Source: CAD feature listing. Evaluate the final solid. Frame: model axes, mm. A direction names the side the tool comes from. Round coordinates to 2 decimals unless told otherwise and drop trailing zeros. Write each loop counter-clockwise with the first axis right and the second up, starting at its lowest first coordinate (ties: lowest second). Pieces come first, ordered by that corner, then holes. Notation, with made-up numbers: (34.25, 50.5) -> (40.25, 50.5) arc R4 cw to (40.25, 56.5) -> close; hole circle Ø7 at (-19.75, -7.75). An arc over 180 degrees is marked (long way). Put each result on its own line as item: value.
```python
from build123d import *

# Parameters (mm, degrees)
PAD_DEPTH        = 11.43
MIRRORED_FACE5_W = 11.43
MIRRORED_FACE5_H = 20.32
PAD001_DEPTH     = 6.85
SKETCH001_W      = 4.191
SKETCH001_H      = 1.778
POCKET_DEPTH     = 10.16
CHAMFER_SIZE     = 1


with BuildPart() as part:
    # Sketch → Pad (new body)
    with BuildSketch(Plane.XZ):
        with BuildLine():
            Line((0, 0), (-10.16, 0))
            add(Edge.make_bspline(
                [(-10.16, 0), (-10.491854, 4.757151), (-8.764645, 7.62), (-8.764645, 7.62)],
                knots=[0, 0, 0, 0, 1, 1, 1, 1], degree=3))
            add(Edge.make_bspline(
                [(-8.764645, 7.62), (-6.92736, 3.81), (0, 3.81)],
                knots=[0, 0, 0, 1, 1, 1], degree=2))
            Line((0, 3.81), (0, 0))
        make_face()
    extrude(amount=PAD_DEPTH)

    # Mirrored: part across YZ


with BuildPart() as part_1:
    add(part.part)
    add(part.part.mirror(Plane.YZ))

    # Mirrored Face5 → Pad001 (add)
    with BuildSketch(Plane(origin=(0, -5.715, 0), x_dir=(0, -1, 0), z_dir=(0, 0, -1))):
        Rectangle(MIRRORED_FACE5_W, MIRRORED_FACE5_H)
    extrude(amount=PAD001_DEPTH)

    # Sketch001 (on Face4 of Pad001) → Pocket (cut)
    with BuildSketch(Plane(origin=(0, 0, -6.85), x_dir=(1, 0, 0), z_dir=(0, 0, -1))):
        with Locations((0, 5.715)):
            Rectangle(SKETCH001_W, SKETCH001_H)
    extrude(amount=-POCKET_DEPTH, mode=Mode.SUBTRACT)

    # Chamfer
    chamfer_edges = [part_1.edges().sort_by_distance(p)[0] for p in [
        (0, 0, -6.85),
        (10.16, -5.715, -6.85),
        (0, -11.43, -6.85),
        (-10.16, -5.715, -6.85),
    ]]
    chamfer(chamfer_edges, length=CHAMFER_SIZE)


solid = part_1.part
```
Q1. Reachability of faces 5 (the flat face through (0, -11.43, -1)), 6 (the flat face through (2.096, -6, -2)), 7 (the flat face through (-10.16, -6, -3)) from +Z, -Z, +X, -X, +Y, -Y: full face, straight path, thin tool, end or side. Return the list, or none.
Ans:
face 5: +Z, -Z, +X, -X, -Y
face 6: -Z
face 7: -Z, -X, +Y, -Y
Q2. Material intervals for line 1 (Y direction, x = 1.25, z = 0.25); line 2 (X direction, y = -3.5, z = -2.25); line 3 (X direction, y = -5, z = 0.5), sorted ascending. Write a range as [from, to].
Ans:
line 1: y = [-11.43, -6.6], [-4.83, 0]
line 2: x = [-10.16, 10.16]
line 3: x = [-10.19, -2.1], [2.1, 10.19]
Q3. Cut plane A-A on z = -2.75. Output: boundary loops of the cut face in (x, y).
Ans:
outline: (-10.16, -11.43) -> (10.16, -11.43) -> (10.16, 0) -> (-10.16, 0) -> close; hole (-2.1, -6.6) -> (2.1, -6.6) -> (2.1, -4.83) -> (-2.1, -4.83) -> close
Q4. Draft query along X for faces 1 (the flat face through (0, 0, -1)), 2 (the flat face through (-2.096, -6, -2)), 3 (the flat face through (0, -4.826, -2)), 4 (the flat face through (10.16, -6, -3)). Return one class per face: +X half, -X half, draft (parallel to the pull), parting line (faces both ways), or undercut.
Ans:
face 1: draft
face 2: undercut
face 3: undercut
face 4: +X half
Q5. Pin query (flat end, axial travel): pin 1 (3 mm diameter, centred on y = -6.5, z = -3, fed in from -X); pin 2 (5 mm diameter, centred on x = -5.5, y = -1.5, fed in from +Z); pin 3 (4 mm diameter, centred on x = -1.5, y = -4.5, fed in from +Z). Return the tip coordinate at first contact, or that it passes through.
Ans:
pin 1: stops at x = -10.16
pin 2: stops at z = 6.44
pin 3: stops at z = 4.11
